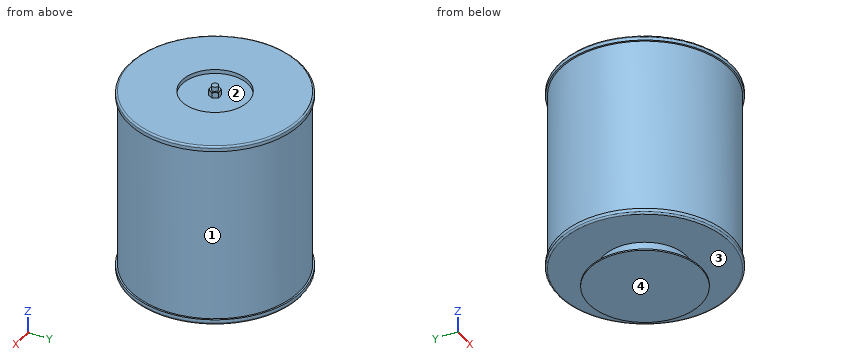
```python
from build123d import *

# Parameters (mm, degrees)
CROQUIS1_R              = 165
SALIENTE_EXTRUIR1_DEPTH = 4
CROQUIS2_R              = 122
SALIENTE_EXTRUIR2_DEPTH = 50
CROQUIS3_R              = 250
SALIENTE_EXTRUIR3_DEPTH = 550
CROQUIS4_R              = 255
SALIENTE_EXTRUIR4_DEPTH = 15
SALIENTE_EXTRUIR5_START = -15
CROQUIS5_R              = 255
SALIENTE_EXTRUIR5_DEPTH = 15
REDONDEO1_R             = 5
CROQUIS6_R              = 98.024692722
CORTAR_EXTRUIR1_DEPTH   = 12
CROQUIS7_R              = 9.525
SALIENTE_EXTRUIR6_DEPTH = 30
SALIENTE_EXTRUIR7_DEPTH = 17
CROQUIS9_R              = 43.133819065
CROQUIS9_R_2            = 14.722431864
CORTAR_EXTRUIR2_DEPTH   = 10
CORTAR_EXTRUIR2_DRAFT   = -55


with BuildPart() as part:
    # Croquis1 → Saliente-Extruir1 (new body)
    with BuildSketch(Plane.XY):
        Circle(CROQUIS1_R)
    extrude(amount=SALIENTE_EXTRUIR1_DEPTH)

    # Croquis2 → Saliente-Extruir2 (add)
    with BuildSketch(Plane.XY.offset(4)):
        Circle(CROQUIS2_R)
    extrude(amount=SALIENTE_EXTRUIR2_DEPTH)

    # Croquis3 → Saliente-Extruir3 (add)
    with BuildSketch(Plane.XY.offset(54)):
        Circle(CROQUIS3_R)
    extrude(amount=SALIENTE_EXTRUIR3_DEPTH)

    # Croquis4 → Saliente-Extruir4 (add)
    with BuildSketch(Plane(origin=(0, 0, 54), x_dir=(-1, 0, 0), z_dir=(0, 0, -1))):
        Circle(CROQUIS4_R)
    extrude(amount=-SALIENTE_EXTRUIR4_DEPTH)

    # Croquis5 → Saliente-Extruir5 (add)
    with BuildSketch(Plane.XY.offset(604).offset(SALIENTE_EXTRUIR5_START)):
        with Locations(Location((0, 0, 0), (0, 0, 180))):
            Circle(CROQUIS5_R)
    extrude(amount=SALIENTE_EXTRUIR5_DEPTH)

    # Redondeo1
    redondeo1_edges = [part.edges().sort_by_distance(p)[0] for p in [
        (255, 0, 54),
        (255, 0, 604),
    ]]
    fillet(redondeo1_edges, radius=REDONDEO1_R)

    # Croquis6 → Cortar-Extruir1 (cut)
    with BuildSketch(Plane.XY.offset(604)):
        Circle(CROQUIS6_R)
    extrude(amount=-CORTAR_EXTRUIR1_DEPTH, mode=Mode.SUBTRACT)

    # Croquis7 → Saliente-Extruir6 (add)
    with BuildSketch(Plane.XY.offset(592)):
        Circle(CROQUIS7_R)
    extrude(amount=SALIENTE_EXTRUIR6_DEPTH)

    # Croquis8 → Saliente-Extruir7 (add)
    with BuildSketch(Plane.XY.offset(592)):
        Polygon((17, 0), (8.5, 14.722431864), (-8.5, 14.722431864), (-17, 0), (-8.5, -14.722431864), (8.5, -14.722431864), align=None)
    extrude(amount=SALIENTE_EXTRUIR7_DEPTH)


with BuildPart() as cortar_extruir2_tool:
    # Croquis9 → Cortar-Extruir2 (with draft: the straight prism first)
    with BuildSketch(Plane.XY.offset(609)):
        Circle(CROQUIS9_R)
        Circle(CROQUIS9_R_2, mode=Mode.SUBTRACT)
    extrude(amount=-CORTAR_EXTRUIR2_DEPTH)
    # Cortar-Extruir2: the draft: its side faces are tilted about the plane it starts from
    cortar_extruir2_sides = [cortar_extruir2_tool.faces().sort_by_distance(p)[0] for p in [
        (-43.133819065, 0, 604),
        (-14.722431864, 0, 604),
    ]]
    draft(cortar_extruir2_sides, Plane.XY.offset(609), CORTAR_EXTRUIR2_DRAFT)


with BuildPart() as part_1:
    add(part.part)

    # Cortar-Extruir2: cut by cortar_extruir2_tool
    add(cortar_extruir2_tool.part, mode=Mode.SUBTRACT)


solid = part_1.part
```
Geometry: final body of the model. Coordinates: model frame, mm. Face numbers are marked on the shaded views. Coordinates: 2 decimals unless noted, no trailing zeros. Order: outer loops, then holes, each group sorted by start corner. A loop starts at its lowest first (then second) coordinate and runs counter-clockwise, first axis right, second up. Notation, with made-up numbers: (40, -27.75) -> (77, -27.75) arc R18 cw to (77, -8.75) -> close; hole circle Ø8 at (23.5, 70.5). An arc over 180 degrees is marked (long way). Answer in a Markdown table with one row per item.
Item 1: Draft query along Z for the marked faces 1, 2, 3 and 4. Return one class per face: released by +Z, released by -Z, zero draft, split by the parting line, or undercut.
Return value:
| item | result |
|---|---|
| face 1 | undercut |
| face 2 | released by +Z |
| face 3 | undercut |
| face 4 | released by -Z |
Item 2: Section A-A on z = 190. Output: boundary loops of the cut face in (x, y).
Return value:
| item | result |
|---|---|
| outline | circle Ø500 at (0, 0) |
Item 3: Ray query, L1, parallel to Y at x = 0, z = 600.25; L2, parallel to Y at x = 0, z = 597.75; L3, parallel to Z at x = -79.5, y = 120. Return the intervals inside material, ascending.
Return value:
| item | result |
|---|---|
| L1 | y = -254.84 to -98.02, -14.72 to 14.72, 98.02 to 254.84 |
| L2 | y = -255 to -98.02, -14.72 to 14.72, 98.02 to 255 |
| L3 | z = 0 to 4, 54 to 604 |
Item 4: Contact query for flat-ended pins moving along their axis: P1, Ø8, axis at x = -172.5, y = 127.5, coming from the -Z side; P2, Ø4, axis at y = -145, z = 270, coming from the -X side; P3, Ø3, axis at x = -152.5, z = 363.5, coming from the -Y side. Output: stop coordinate, or through.
Return value:
| item | result |
|---|---|
| P1 | stops at z = 54 |
| P2 | stops at x = -205.06 |
| P3 | stops at y = -199.25 |
